Geometry check sheet. Reference: the model listing, model coordinates, mm. A direction names the side the tool comes from. Coordinates: 2 decimals unless noted, no trailing zeros. Order: outer loops, then holes, each group sorted by start corner. A loop starts at its lowest first (then second) coordinate and runs counter-clockwise, first axis right, second up. Notation, with made-up numbers: (-18.5, 89) - (27.5, 89) arc R16 cw to (27.5, 94) - close; hole circle Ø6 at (25.25, 27). An arc over 180 degrees is marked (long way). Use CSV: the item, a comma, the result in double quotes. Start each with the question number.
1) Sectioned sample at C-C, the plane y = 2. Record the cut outline in (x, z).
2) Depth check by flat-ended pin: P1, Ø3, axis at y = 8, z = -21, coming from the +X side; P2, Ø6.5, axis at x = 20.5, y = 7.5, coming from the -Z side; P3, Ø5, axis at y = 11, z = -18.5, coming from the -X side; P4, Ø2, axis at y = 7.94, z = -21.55, coming from the +X side. Enter the tip coordinate at first touch or a pass-through.
3) Sectioned sample at B-B, the plane z = -16.5. Record the cut outline in (x, y) (1 decimal).
4) Sectioned sample at A-A, the plane x = 3.5. Record the cut outline in (y, z) (1 decimal).
5) Tool access check on faces 5 (the cylindrical face through (-15.83, 9.46, -1.67)), 6 (the flat face through (-7.671, 5, -22)), 7 (the flat face through (0.317, 8, -24)), 8 (the flat face through (0, 0, -5)). Record the directions out of +Z, -Z, +X, -X, +Y, -Y that give a thin tool (end or side, any length) a straight path to the whole face; none if there is none.
6) Draft check along X on faces 1 (the flat face through (-11.837, 8, -16)), 2 (the cylindrical face through (5.558, 8.013, -23.277)), 3 (the flat face through (-1.207, 7.8, -24.3)), 4 (the flat face through (10.947, 8, -18)). Enter one of: released by +X, released by -X, zero draft, split by the parting line, or undercut.
7) Thickness scan on probe 1 along X at (y, z) = (0.75, -20); probe 2 along Y at (x, z) = (18.5, 5.5) (3 decimals); probe 3 along X at (y, z) = (9, 0.5). Record the ranges inside material, lowest first. Write a range as [from, to].
8) Sectioned sample at D-D, the plane x = -19.5. Record the cut outline in (y, z) (3 decimals), and give its area (3 significant figures).
from build123d import *

# Parameters (mm, degrees)
BOSS_EXTRUDE1_DEPTH                            = 15.875
F_8_32_TAPPED_HOLE1_D                          = 3.4544
F_8_32_TAPPED_HOLE1_DEPTH                      = 10.6299
CBORE_FOR_8_SOCKET_HEAD_CAP_SCREW1_D           = 4.9149
CBORE_FOR_8_SOCKET_HEAD_CAP_SCREW1_DEPTH       = 10.6299
CBORE_FOR_8_SOCKET_HEAD_CAP_SCREW1_CBORE_D     = 7.9375
CBORE_FOR_8_SOCKET_HEAD_CAP_SCREW1_CBORE_DEPTH = 4.1656
CBORE_FOR_8_SOCKET_HEAD_CAP_SCREW2_D           = 4.9149
CBORE_FOR_8_SOCKET_HEAD_CAP_SCREW2_CBORE_D     = 7.9375
CBORE_FOR_8_SOCKET_HEAD_CAP_SCREW2_CBORE_DEPTH = 10.5156


with BuildPart() as part:
    # Sketch1 → Boss-Extrude1 (new body)
    with BuildSketch(Plane(origin=(0, 0, 0), x_dir=(1, 0, 0), z_dir=(0, 1, 0))):
        with BuildLine():
            Line((-11.836826281, 27.901732418), (-1.206926281, 27.901732418))
            Line((-1.206926281, 27.901732418), (-1.206926281, 18.554532418))
            ThreePointArc((-1.206926281, 18.554532418), (-0.444926281, 5.900418206), (0.317073719, 18.554532418))
            Line((0.317073719, 18.554532418), (0.317073719, 27.901732418))
            Line((0.317073719, 27.901732418), (10.946973719, 27.901732418))
            Line((10.946973719, 27.901732418), (10.946973719, 8.657386186))
            Line((10.946973719, 8.657386186), (24.955073719, 2.526772877))
            Line((24.955073719, 2.526772877), (24.955073719, -9.690267582))
            Line((24.955073719, -9.690267582), (-25.844926281, -9.690267582))
            Line((-25.844926281, -9.690267582), (-25.844926281, 2.526772877))
            Line((-25.844926281, 2.526772877), (-11.836826281, 8.657386186))
            Line((-11.836826281, 8.657386186), (-11.836826281, 27.901732418))
        make_face()
    extrude(amount=BOSS_EXTRUDE1_DEPTH)

    # #8-32 Tapped Hole1
    with Locations(Plane(origin=(10.946973719, 0, 0), x_dir=(0, 0, -1), z_dir=(1, 0, 0))):
        with Locations((21.551732418, 7.9375)):
            Hole(F_8_32_TAPPED_HOLE1_D / 2, depth=F_8_32_TAPPED_HOLE1_DEPTH)

    # CBORE for #8 Socket Head Cap Screw1
    with Locations(Plane.ZY.offset(11.836826281)):
        with Locations((-21.551732418, 7.9375)):
            CounterBoreHole(CBORE_FOR_8_SOCKET_HEAD_CAP_SCREW1_D / 2, CBORE_FOR_8_SOCKET_HEAD_CAP_SCREW1_CBORE_D / 2, CBORE_FOR_8_SOCKET_HEAD_CAP_SCREW1_CBORE_DEPTH, depth=CBORE_FOR_8_SOCKET_HEAD_CAP_SCREW1_DEPTH)

    # CBORE for #8 Socket Head Cap Screw2 (through all)
    with Locations(Plane(origin=(0, 0, -8.657386186), x_dir=(1, 0, 0), z_dir=(0, 0, -1))):
        with Locations((18.605073719, -7.9375), (-19.494926281, -7.9375)):
            CounterBoreHole(CBORE_FOR_8_SOCKET_HEAD_CAP_SCREW2_D / 2, CBORE_FOR_8_SOCKET_HEAD_CAP_SCREW2_CBORE_D / 2, CBORE_FOR_8_SOCKET_HEAD_CAP_SCREW2_CBORE_DEPTH)


solid = part.part
Evaluation:
1,outline,"(-25.84, -2.53) - (-11.84, -8.66) - (-11.84, -27.9) - (-1.21, -27.9) - (-1.21, -18.55) arc R6.35 cw (long way) to (0.32, -18.55) - (0.32, -27.9) - (10.95, -27.9) - (10.95, -8.66) - (24.96, -2.53) - (24.96, 9.69) - (-25.84, 9.69) - close"
2,P1,"x = 10.95"
2,P2,"z = -4.64"
2,P3,"x = -11.84"
2,P4,"through"
3,outline,"(-11.8, 0) - (-5.2, 0) - (-5.2, 15.9) - (-11.8, 15.9) - close; (4.3, 0) - (10.9, 0) - (10.9, 15.9) - (4.3, 15.9) - close"
4,outline,"(0, -27.9) - (15.9, -27.9) - (15.9, -17.2) - (0, -17.2) - close; (0, -7.3) - (15.9, -7.3) - (15.9, 9.7) - (0, 9.7) - close; hole circle Ø3.5 at (7.9, -21.6)"
5,face 5,"-Z"
5,face 6,"-X"
5,face 7,"-Z, +Y, -Y"
5,face 8,"+Z, -Z, +X, -X, -Y"
6,face 1,"released by -X"
6,face 2,"zero draft"
6,face 3,"undercut"
6,face 4,"released by +X"
7,probe 1,"[-11.84, -1.21], [0.32, 10.95]"
7,probe 2,"[0, 5.482], [10.393, 15.875]"
7,probe 3,"[-25.84, -23.32], [-15.67, 14.78], [22.43, 24.96]"
8,outline,"(0, -5.304) - (3.969, -5.304) - (3.969, 1.858) - (5.48, 1.858) - (5.48, 9.69) - (0, 9.69) - close; (10.395, 1.858) - (11.906, 1.858) - (11.906, -5.304) - (15.875, -5.304) - (15.875, 9.69) - (10.395, 9.69) - close"
8,area,"143 mm²"
